```python
from build123d import *

# Parameters (mm, degrees)
SKETCH_1_W          = 330
SKETCH_1_H          = 100
EXTRUDE_1_DEPTH     = 5
SKETCH_3_R          = 1.515
CUT_EXTRUDE_1_DEPTH = 259.310540517
SKETCH_4_R          = 1.05
CUT_EXTRUDE_2_DEPTH = 259.310540517


with BuildPart() as part:
    # 草图1 → 凸台-拉伸1 (new body)
    with BuildSketch(Plane(origin=(0, 0, 0), x_dir=(1, 0, 0), z_dir=(0, 1, 0))):
        with Locations((9.630350195, -140.272373541)):
            Rectangle(SKETCH_1_W, SKETCH_1_H)
    extrude(amount=EXTRUDE_1_DEPTH)

    # 草图3 → 切除-拉伸1 (cut, through all)
    with BuildSketch(Plane(origin=(0, 5, 0), x_dir=(1, 0, 0), z_dir=(0, 1, 0))):
        with Locations(Location((-2.369649805, -97.272373541, 0), (0, 0, 270))):
            Circle(SKETCH_3_R)
        with Locations(Location((21.630350195, -97.272373541, 0), (0, 0, 90))):
            Circle(SKETCH_3_R)
        with Locations(Location((-2.369649805, -115.272373541, 0), (0, 0, 270))):
            Circle(SKETCH_3_R)
        with Locations(Location((21.630350195, -115.272373541, 0), (0, 0, 90))):
            Circle(SKETCH_3_R)
    extrude(amount=-CUT_EXTRUDE_1_DEPTH, mode=Mode.SUBTRACT)

    # 草图4 → 切除-拉伸2 (cut, through all)
    with BuildSketch(Plane(origin=(0, 5, 0), x_dir=(1, 0, 0), z_dir=(0, 1, 0))):
        with Locations(Location((-140.369649805, -170.272373541, 0), (0, 0, 270))):
            Circle(SKETCH_4_R)
        with Locations(Location((-140.369649805, -130.272373541, 0), (0, 0, 90))):
            Circle(SKETCH_4_R)
        with Locations(Location((-98.369649805, -170.272373541, 0), (0, 0, 270))):
            Circle(SKETCH_4_R)
        with Locations(Location((-98.369649805, -130.272373541, 0), (0, 0, 90))):
            Circle(SKETCH_4_R)
        with Locations(Location((117.630350195, -130.272373541, 0), (0, 0, 270))):
            Circle(SKETCH_4_R)
        with Locations(Location((117.630350195, -170.272373541, 0), (0, 0, 90))):
            Circle(SKETCH_4_R)
        with Locations(Location((159.630350195, -130.272373541, 0), (0, 0, 270))):
            Circle(SKETCH_4_R)
        with Locations(Location((159.630350195, -170.272373541, 0), (0, 0, 90))):
            Circle(SKETCH_4_R)
        with BuildLine():
            Line((-10.369649805, -142.272373541), (29.630350195, -142.272373541))
            ThreePointArc((29.630350195, -142.272373541), (37.630350195, -150.272373541), (29.630350195, -158.272373541))
            Line((29.630350195, -158.272373541), (-10.369649805, -158.272373541))
            ThreePointArc((-10.369649805, -158.272373541), (-18.369649805, -150.272373541), (-10.369649805, -142.272373541))
        make_face()
    extrude(amount=-CUT_EXTRUDE_2_DEPTH, mode=Mode.SUBTRACT)


solid = part.part
```
Part model, mm, in its own coordinate system. A direction names the side the tool comes from. Give positions to 0.01 mm unless a question says otherwise; leave off trailing zeros. Write each loop counter-clockwise with the first axis right and the second up, starting at its lowest first coordinate (ties: lowest second). Pieces come first, ordered by that corner, then holes. Notation, with made-up numbers: (39.25, -10) -> (49.25, -10) arc R14 cw to (49.25, 1) -> close; hole circle Ø10 at (28.25, 61). An arc over 180 degrees is marked (long way). Put each result on its own line as item: value. Start each with the question number.
Item 1: Cut at B-B (y = 4). State how many separate pieces and enclosed holes the cut face has, then the cut area to 3 significant figures.
Item 2: Wall check: L1, parallel to X at y = 3.3, z = 96; L2, parallel to X at y = 4.5, z = 145; L3, parallel to X at y = 3.2, z = 147. Give the ranges that are in metal, low to high. Write a range as [from, to].
Item 3: Cut at A-A (z = 154.5). List the corners of the cut face in (x, y), then the cut area to 3 significant figures.
Item 4: Pull direction Z, two halves, no side cores. Call faces 1 (the face through (-18.368, 2.535, 150.448)), 2 (the face through (7, 5, 140)): pulls with the +Z half, pulls with the -Z half, needs draft (parallel to the pull), parting line crosses it, or undercut.
Item 5: Pin check, flat tip, straight feed: pin 1 Ø1.3 at (x, z) = (-98.37, 130.27) entering from +Y. Stop position of the tip, or through.
Item 6: Which spindle directions (+Z, -Z, +X, -X, +Y, -Y) get a long thin tool onto all of the face, cutting with end or side? Do faces 3 (the face through (37.63, 2.54, 150.1)), 4 (the face through (7, 0, 140)). Say none if no direction does.
Answer list:
1. separate pieces: 1
1. enclosed holes: 13
1. area: 32,100 mm2
2. L1: x = [-155.37, -3.19], [-1.55, 20.81], [22.45, 174.63]
2. L2: x = [-155.37, -16.39], [35.65, 174.63]
2. L3: x = [-155.37, -17.67], [36.93, 174.63]
3. outline: (-155.37, 0) -> (-17.16, 0) -> (-17.16, 5) -> (-155.37, 5) -> close; (36.42, 0) -> (174.63, 0) -> (174.63, 5) -> (36.42, 5) -> close
3. area: 1,380 mm2
4. face 1: undercut
4. face 2: needs draft
5. pin 1: passes through
6. face 3: +Y, -Y
6. face 4: +Z, -Z, +X, -X, -Y
